Could you check a few things on this model? Use its own coordinates, in mm. Face numbers are marked on the shaded views. A direction names the side the tool comes from. Give positions to 0.01 mm unless a question says otherwise; leave off trailing zeros. Order: outer loops, then holes, each group sorted by start corner. A loop starts at its lowest first (then second) coordinate and runs counter-clockwise, first axis right, second up. Notation, with made-up numbers: M 33.25,33 L 40.25,33 A25 cw 40.25,63 Z; hole C 30.5,31 d2. An arc over 180 degrees is marked long. Use a Markdown table: item, result. Add a question column.
```python
from build123d import *

# Parameters (mm, degrees)
F1_DEPTH = 2
F2_DEPTH = 19
F3_R     = 2.75
F3_R_2   = 1.25
F4_DEPTH = 5
F5_W     = 9
F5_H     = 2
F5_W_2   = 17
F5_W_3   = 8
F5_W_4   = 2
F5_H_2   = 15.1
F5_H_3   = 15.9
F6_DEPTH = 12
F7_W     = 15.6
F7_H     = 4
F8_DEPTH = 5
F9_R     = 2.5


with BuildPart() as f1:
    # F0 (on Top) → F1 (new body)
    with BuildSketch(Plane.XY):
        with BuildLine():
            ThreePointArc((0, 2.5), (0.732233047, 0.732233047), (2.5, 0))
            Line((2.5, 0), (88.5, 0))
            ThreePointArc((88.5, 0), (90.267766953, 0.732233047), (91, 2.5))
            Line((91, 2.5), (91, 59.5))
            ThreePointArc((91, 59.5), (90.267766953, 61.267766953), (88.5, 62))
            Line((88.5, 62), (2.5, 62))
            ThreePointArc((2.5, 62), (0.732233047, 61.267766953), (0, 59.5))
            Line((0, 59.5), (0, 2.5))
        make_face()
        with BuildLine():
            ThreePointArc((2, 59.5), (2.1464466094, 59.8535533906), (2.5, 60))
            Line((2.5, 60), (88.5, 60))
            ThreePointArc((88.5, 60), (88.8535533906, 59.8535533906), (89, 59.5))
            Line((89, 59.5), (89, 2.5))
            ThreePointArc((89, 2.5), (88.8535533906, 2.1464466094), (88.5, 2))
            Line((88.5, 2), (2.5, 2))
            ThreePointArc((2.5, 2), (2.1464466094, 2.1464466094), (2, 2.5))
            Line((2, 2.5), (2, 59.5))
        make_face(mode=Mode.SUBTRACT)
        with BuildLine():
            Line((88.5, 60), (2.5, 60))
            ThreePointArc((2.5, 60), (2.1464466094, 59.8535533906), (2, 59.5))
            Line((2, 59.5), (2, 2.5))
            ThreePointArc((2, 2.5), (2.1464466094, 2.1464466094), (2.5, 2))
            Line((2.5, 2), (88.5, 2))
            ThreePointArc((88.5, 2), (88.8535533906, 2.1464466094), (89, 2.5))
            Line((89, 2.5), (89, 59.5))
            ThreePointArc((89, 59.5), (88.8535533906, 59.8535533906), (88.5, 60))
        make_face()
    extrude(amount=F1_DEPTH)

    # F0 (on Top) → F2 (join)
    with BuildSketch(Plane.XY):
        with BuildLine():
            ThreePointArc((0, 2.5), (0.732233047, 0.732233047), (2.5, 0))
            Line((2.5, 0), (88.5, 0))
            ThreePointArc((88.5, 0), (90.267766953, 0.732233047), (91, 2.5))
            Line((91, 2.5), (91, 59.5))
            ThreePointArc((91, 59.5), (90.267766953, 61.267766953), (88.5, 62))
            Line((88.5, 62), (2.5, 62))
            ThreePointArc((2.5, 62), (0.732233047, 61.267766953), (0, 59.5))
            Line((0, 59.5), (0, 2.5))
        make_face()
        with BuildLine():
            ThreePointArc((2, 59.5), (2.1464466094, 59.8535533906), (2.5, 60))
            Line((2.5, 60), (88.5, 60))
            ThreePointArc((88.5, 60), (88.8535533906, 59.8535533906), (89, 59.5))
            Line((89, 59.5), (89, 2.5))
            ThreePointArc((89, 2.5), (88.8535533906, 2.1464466094), (88.5, 2))
            Line((88.5, 2), (2.5, 2))
            ThreePointArc((2.5, 2), (2.1464466094, 2.1464466094), (2, 2.5))
            Line((2, 2.5), (2, 59.5))
        make_face(mode=Mode.SUBTRACT)
    extrude(amount=F2_DEPTH)

    # F3 (on face) → F4 (join)
    with BuildSketch(Plane.XY.offset(2)):
        with Locations((6.5, 55.5)):
            Circle(F3_R)
        with Locations((6.5, 55.5)):
            Circle(F3_R_2, mode=Mode.SUBTRACT)
        with Locations((64.5, 55.5)):
            Circle(F3_R)
        with Locations((64.5, 55.5)):
            Circle(F3_R_2, mode=Mode.SUBTRACT)
        with Locations((6.5, 6.5)):
            Circle(F3_R)
        with Locations((6.5, 6.5)):
            Circle(F3_R_2, mode=Mode.SUBTRACT)
        with Locations((64.5, 6.5)):
            Circle(F3_R)
        with Locations((64.5, 6.5)):
            Circle(F3_R_2, mode=Mode.SUBTRACT)
    extrude(amount=F4_DEPTH)

    # F5 (on face) → F6 (cut)
    with BuildSketch(Plane.XY.offset(19)):
        with Locations((13.55, 1)):
            Rectangle(F5_W, F5_H)
        with Locations((35, 1)):
            Rectangle(F5_W_2, F5_H)
        with Locations((57.25, 1)):
            Rectangle(F5_W_3, F5_H)
        with Locations((90, 49.95)):
            Rectangle(F5_W_4, F5_H_2)
        with Locations((90, 30.95)):
            Rectangle(F5_W_4, F5_H_2)
        with Locations((90, 13.25)):
            Rectangle(F5_W_4, F5_H_3)
    extrude(amount=-F6_DEPTH, mode=Mode.SUBTRACT)

    # F7 (on face) → F8 (cut)
    with BuildSketch(Plane(origin=(0, 0, 0), x_dir=(0, -1, 0), z_dir=(-1, 0, 0))):
        with Locations((-31.7, 6)):
            Rectangle(F7_W, F7_H)
    extrude(amount=-F8_DEPTH, mode=Mode.SUBTRACT)

    # F9
    f9_edges = [f1.edges().sort_by_distance(p)[0] for p in [
        (45.5, 0, 0),
    ]]
    fillet(f9_edges, radius=F9_R)


solid = f1.part
```
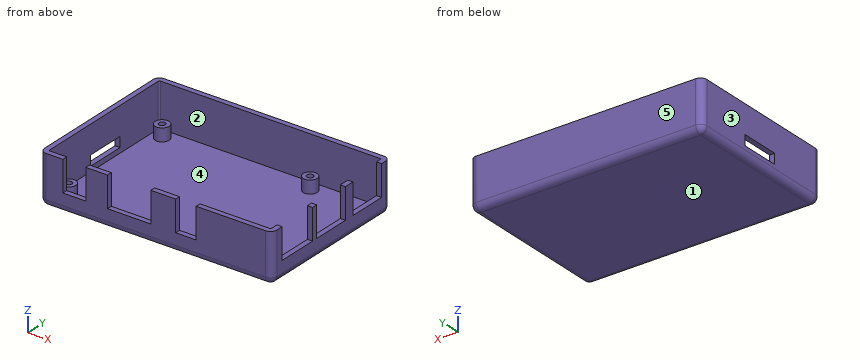
1) We'd pull the mould along X, two halves only. Please class the marked faces 1, 2 and 3: pulls with the +X half, pulls with the -X half, needs draft (parallel to the pull), parting line crosses it, or undercut.
2) For the marked faces 4 and 5, which set-ups out of +Z, -Z, +X, -X, +Y, -Y let a thin tool reach every point of the face, with its end or its side?
3) Suppose I cut it at B-B on y = 6.5. Please give me the cut outline in (x, z).
4) For pin 1 (2 mm diameter, centred on x = 7, y = 55, fed in from +Z); pin 2 (0.6 mm diameter, centred on x = 1, y = 28, fed in from -Z); pin 3 (1 mm diameter, centred on y = 1, z = 14, fed in from +X); pin 4 (8 mm diameter, centred on x = 40.5, z = 16, fed in from -Y), each with a flat end and sliding along its axis, tell me the tip position at first contact or that it passes through.
5) Please list where these lines run through material, in increasing order: line 1 (Y direction, x = 6.5, z = 4.75); line 2 (Y direction, x = 56, z = 6); line 3 (X direction, y = 4, z = 4). Write a range as from..to.
6) Suppose I cut it at A-A on z = 5.25. Count the separate pieces of the cut face and the enclosed holes in it, and give its area (3 significant figures).
7) Suppose I cut it at C-C on x = 75. Please give me the cut outline in (y, z).
Values found:
| question | item | result |
|---|---|---|
| 1 | face 1 | needs draft |
| 1 | face 2 | undercut |
| 1 | face 3 | pulls with the -X half |
| 2 | face 4 | +Z |
| 2 | face 5 | +Z, -Z, +X, -X, +Y |
| 3 | outline | M 0,2.5 A2.5 ccw 2.5,0 L 88.5,0 A2.5 ccw 91,2.5 L 91,7 L 89,7 L 89,2 L 67.25,2 L 67.25,7 L 65.75,7 L 65.75,2 L 63.25,2 L 63.25,7 L 61.75,7 L 61.75,2 L 9.25,2 L 9.25,7 L 7.75,7 L 7.75,2 L 5.25,2 L 5.25,7 L 3.75,7 L 3.75,2 L 2,2 L 2,19 L 0,19 Z |
| 4 | pin 1 | stops at z = 7 |
| 4 | pin 2 | stops at z = 0.31 |
| 4 | pin 3 | stops at x = 90.79 |
| 4 | pin 4 | stops at y = 0 |
| 5 | line 1 | y = 0..2, 3.75..5.25, 7.75..9.25, 52.75..54.25, 56.75..58.25, 60..62 |
| 5 | line 2 | y = 0..2, 60..62 |
| 5 | line 3 | x = 0..2, 5.35..7.65, 63.35..65.65, 89..91 |
| 6 | separate pieces | 5 |
| 6 | enclosed holes | 4 |
| 6 | area | 635 mm^2 |
| 7 | outline | M 0,2.5 A2.5 ccw 2.5,0 L 59.5,0 A2.5 ccw 62,2.5 L 62,19 L 60,19 L 60,2 L 2,2 L 2,19 L 0,19 Z |
